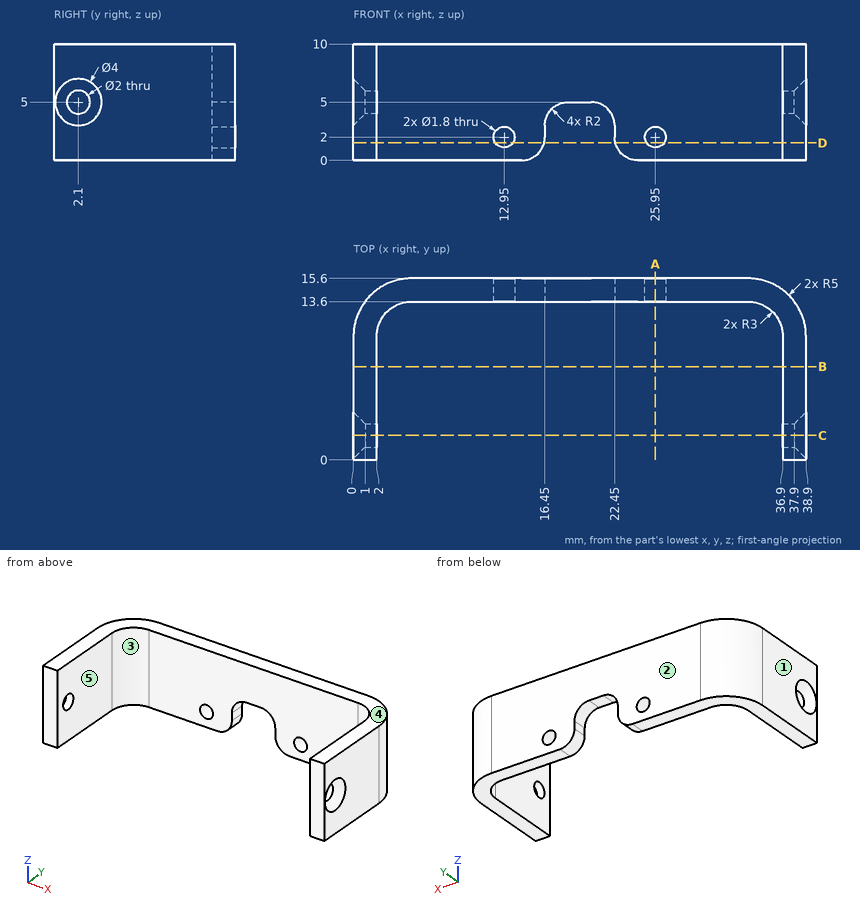
Design review of the part shown in the three views and the two pictorial views. Dimensions are in mm from the part's minimum x, y and z. A direction names the side the tool comes from. Coordinates: 2 decimals unless noted, no trailing zeros. Loops run counter-clockwise (first coordinate to the right, second up) from the corner with the lowest first, then second, coordinate; pieces in that order, holes last. Notation, with made-up numbers: (29, -1) -> (68, -1) arc R20 cw to (68, 12) -> close; hole circle Ø4 at (32.5, 25). An arc over 180 degrees is marked (long way). Answer as CSV lines item,"result".
Item 1: Take a section at C-C, the plane y = 2.1. State the section outline as (x, z) points.
Results below:
outline,"(0, 0) -> (2, 0) -> (2, 4) -> (1, 4) -> (0, 3) -> close; (0, 7) -> (1, 6) -> (2, 6) -> (2, 10) -> (0, 10) -> close; (36.9, 0) -> (38.9, 0) -> (38.9, 3) -> (37.9, 4) -> (36.9, 4) -> close; (36.9, 6) -> (37.9, 6) -> (38.9, 7) -> (38.9, 10) -> (36.9, 10) -> close"
Item 2: Take a section at B-B, the plane y = 8. State the section outline as (x, z) points, and give its area (3 significant figures).
Results below:
outline,"(0, 0) -> (2, 0) -> (2, 10) -> (0, 10) -> close; (36.9, 0) -> (38.9, 0) -> (38.9, 10) -> (36.9, 10) -> close"
area,"40.0 mm2"
Item 3: For L1, parallel to X at y = 9.25, z = 9.25; L2, parallel to Y at x = 1.8, z = 5; L3, parallel to Y at x = 12.5, z = 6.5, list the stretches that pass through material, from the lowest coordinate up.
Results below:
L1,"x = 0 to 2, 36.9 to 38.9"
L2,"y = 0 to 1.1, 3.1 to 14.44"
L3,"y = 13.6 to 15.6"
Item 4: Insertion check: pin 1 (4 mm diameter, centred on x = 12, z = 8.5, fed in from -Y); pin 2 (2.5 mm diameter, centred on y = 2.1, z = 5, fed in from -X); pin 3 (1.1 mm diameter, centred on y = 14.5, z = 2.5, fed in from +X); pin 4 (1.8 mm diameter, centred on y = 2.1, z = 5, fed in from +X). Each pin has a flat end and moves straight along its axis. Give the tip position at first contact, or say it passes through.
Results below:
pin 1,"stops at y = 13.6"
pin 2,"stops at x = 0.75"
pin 3,"stops at x = 37.61"
pin 4,"passes through"
Item 5: Take a section at D-D, the plane z = 1.5. State the section outline as (x, y) points, and give its area (3 significant figures).
Results below:
outline,"(0, 0) -> (2, 0) -> (2, 10.6) arc R3 cw to (5, 13.6) -> (12.2, 13.6) -> (12.2, 15.6) -> (5, 15.6) arc R5 ccw to (0, 10.6) -> close; (13.7, 13.6) -> (16.39, 13.6) -> (16.39, 15.6) -> (13.7, 15.6) -> close; (22.51, 13.6) -> (25.2, 13.6) -> (25.2, 15.6) -> (22.51, 15.6) -> close; (26.7, 13.6) -> (33.9, 13.6) arc R3 cw to (36.9, 10.6) -> (36.9, 0) -> (38.9, 0) -> (38.9, 10.6) arc R5 ccw to (33.9, 15.6) -> (26.7, 15.6) -> close"
area,"107 mm2"
Item 6: Machinability: for the marked faces 4 and 5, which of the approach directions +Z, -Z, +X, -X, +Y, -Y give a long, thin tool a straight path to every point of the face, cutting with its end or side? Answer none if there is none.
Results below:
face 4,"+Z, +X, -X, +Y, -Y"
face 5,"+Z, -Z, -Y"
Item 7: Take a section at A-A, the plane x = 25.95. State the section outline as (y, z) points, and give its area (3 significant figures).
Results below:
outline,"(13.6, 0) -> (15.6, 0) -> (15.6, 1.1) -> (13.6, 1.1) -> close; (13.6, 2.9) -> (15.6, 2.9) -> (15.6, 10) -> (13.6, 10) -> close"
area,"16.4 mm2"
Item 8: Draft analysis for pull direction X (two halves, no side actions). For the marked faces 1, 2 and 3, state which applies: +X half, -X half, draft (parallel to the pull), parting line (faces both ways), or undercut.
Results below:
face 1,"-X half"
face 2,"draft"
face 3,"undercut"
